Can you work these out from the model? Positions are in its coordinate system, mm. Face numbers are marked on the shaded views. A direction names the side the tool comes from. Coordinates: 2 decimals unless noted, no trailing zeros. Loops run counter-clockwise (first coordinate to the right, second up) from the corner with the lowest first, then second, coordinate; pieces in that order, holes last. Notation, with made-up numbers: (26.5, 51.5) -> (60.5, 51.5) arc R26 ccw to (60.5, 82.5) -> close; hole circle Ø10 at (12.25, -30.5). An arc over 180 degrees is marked (long way). Use one line per item in the form item = value. Start each with the question number.
(1) Imagine slicing it at C-C (z = 14). List the corners of the cut face in (x, y) for me.
(2) Thinking about a two-plate mould opening in X: for the marked faces 4, 5, 6 and 7, which applies, released by +X, released by -X, zero draft, split by the parting line, or undercut?
(3) Imagine slicing it at D-D (y = -24). List the corners of the cut face in (x, z) for me, plus the area to 3 significant figures.
(4) On a 3-axis mill with a long thin cutter (end or side, diameter ignored), from which of +Z, -Z, +X, -X, +Y, -Y can I reach the whole of each face in a straight line? I mean the marked faces 1, 2 and 3. Say none if no direction works.
(5) I'm going to push a flat-ended pin straight in: pin 1 (10 mm diameter, centred on x = -2.5, y = -18.5, fed in from +Z). Where does the tip first touch, or does it pass through?
(6) Imagine slicing it at A-A (z = 44). List the corners of the cut face in (x, y) for me, plus the area to 3 significant figures.
(7) I need wall thicknesses on line 1 (X direction, y = 36, z = 26); line 2 (Y direction, x = 0, z = 23). Which ranges of each line are inside material? Lowest first, please. Write a range as [from, to].
```python
from build123d import *

# Parameters (mm, degrees)
ESQUISSE1_W        = 96
ESQUISSE1_H        = 96
ESQUISSE1_W_2      = 80
ESQUISSE1_H_2      = 80
BOSS_EXTRU_1_DEPTH = 48
ESQUISSE2_W        = 96
ESQUISSE2_H        = 96
BOSS_EXTRU_3_DEPTH = 10
ESQUISSE3_R        = 16
BOSS_EXTRU_4_DEPTH = 12.5
ESQUISSE4_R        = 18.5
ESQUISSE4_R_2      = 11.5
BOSS_EXTRU_5_DEPTH = 48
CHANFREIN1_SIZE2   = 48
CHANFREIN1_SIZE    = 4.199455849


with BuildPart() as part:
    # Esquisse1 → Boss.-Extru.1 (new body)
    with BuildSketch(Plane.XY):
        Rectangle(ESQUISSE1_W, ESQUISSE1_H)
        Rectangle(ESQUISSE1_W_2, ESQUISSE1_H_2, mode=Mode.SUBTRACT)
    extrude(amount=BOSS_EXTRU_1_DEPTH)

    # Esquisse2 → Boss.-Extru.3 (add)
    with BuildSketch(Plane.XY.offset(48)):
        Rectangle(ESQUISSE2_W, ESQUISSE2_H)
    extrude(amount=BOSS_EXTRU_3_DEPTH)

    # Esquisse3 → Boss.-Extru.4 (add)
    with BuildSketch(Plane.XY.offset(58)):
        with Locations(Location((-24, 24, 0), (0, 0, 180))):
            Circle(ESQUISSE3_R)
        with Locations(Location((24, 24, 0), (0, 0, 180))):
            Circle(ESQUISSE3_R)
        with Locations(Location((24, -24, 0), (0, 0, 180))):
            Circle(ESQUISSE3_R)
        with Locations(Location((-24, -24, 0), (0, 0, 180))):
            Circle(ESQUISSE3_R)
    extrude(amount=BOSS_EXTRU_4_DEPTH)

    # Esquisse4 → Boss.-Extru.5 (add)
    with BuildSketch(Plane(origin=(0, 0, 0), x_dir=(-1, 0, 0), z_dir=(0, 0, -1))):
        Circle(ESQUISSE4_R)
        Circle(ESQUISSE4_R_2, mode=Mode.SUBTRACT)
    extrude(amount=-BOSS_EXTRU_5_DEPTH)

    # Chanfrein1
    chanfrein1_edges = [part.edges().sort_by_distance(p)[0] for p in [
        (18.5, 0, 48),
    ]]
    chanfrein1_side = [part.faces().sort_by_distance(p)[0] for p in [
        (18.583989117, 0, 48),
    ]]
    chamfer(chanfrein1_edges, length=CHANFREIN1_SIZE - 0.0001, length2=CHANFREIN1_SIZE2 - 0.0001, reference=chanfrein1_side[0])  # a hair under: the kernel refuses the full size


solid = part.part
```
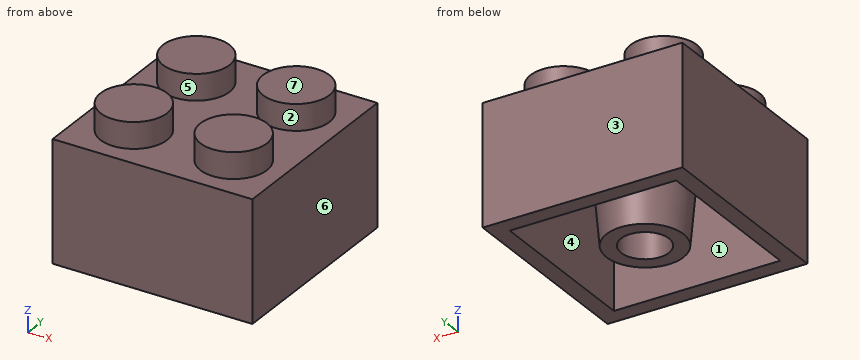
Worked out:
q1.outline = (-48, -48) -> (48, -48) -> (48, 48) -> (-48, 48) -> close; circle Ø39.45 at (0, 0); hole (-40, -40) -> (40, -40) -> (40, 40) -> (-40, 40) -> close; hole circle Ø23 at (0, 0)
q2.face_4 = undercut
q2.face_5 = undercut
q2.face_6 = released by +X
q2.face_7 = zero draft
q3.outline = (-48, 0) -> (-40, 0) -> (-40, 48) -> (40, 48) -> (40, 0) -> (48, 0) -> (48, 58) -> (40, 58) -> (40, 70.5) -> (8, 70.5) -> (8, 58) -> (-8, 58) -> (-8, 70.5) -> (-40, 70.5) -> (-40, 58) -> (-48, 58) -> close
q3.area = 2,530 mm2
q4.face_1 = -Z
q4.face_2 = +Z
q4.face_3 = +Z, -Z, +X, -X, +Y
q5.pin_1 = 58
q6.outline = (-48, -48) -> (48, -48) -> (48, 48) -> (-48, 48) -> close; circle Ø44.7 at (0, 0); hole (-40, -40) -> (40, -40) -> (40, 40) -> (-40, 40) -> close; hole circle Ø23 at (0, 0)
q6.area = 3,970 mm2
q7.line_1 = [-48, -40], [40, 48]
q7.line_2 = [-48, -40], [-20.51, -11.5], [11.5, 20.51], [40, 48]
